The model under review builds one solid part; all positions refer to its coordinate system, in mm. Face numbers are marked on the shaded views. A direction names the side the tool comes from. Coordinates: 2 decimals unless noted, no trailing zeros. Write each loop counter-clockwise with the first axis right and the second up, starting at its lowest first coordinate (ties: lowest second). Pieces come first, ordered by that corner, then holes.
1) Mouldability with a two-part tool opening along X and no side actions: class the marked faces 1, 2, 3 and 4 as released by +X, released by -X, zero draft, split by the parting line, or undercut.
2) Machinability: for the marked faces 5 and 6, which of the approach directions +Z, -Z, +X, -X, +Y, -Y give a long, thin tool a straight path to every point of the face, cutting with its end or side? Answer none if there is none.
3) For line 1 (X direction, y = 20, z = 32); line 2 (Z direction, x = 57.5, y = 20.5); line 3 (Z direction, x = 3, y = 8.25), list the stretches that pass through material, from the lowest coordinate up.
4) Add section B-B, the plane y = 19.25. State the section outline as (x, z) points.
5) Add section C-C, the plane x = 40.5. State the section outline as (y, z) points.
6) Add section A-A, the plane x = 13.5. State the section outline as (y, z) points, then the cut area to 3 significant figures.
7) For P1, Ø10, axis at x = -8, y = 21.5, coming from the +Z side; P2, Ø2, axis at x = -6, y = 17, coming from the -Z side; P3, Ø6, axis at x = -37.69, z = -47.06, coming from the -Y side; P4, Ø0.5, axis at x = -2, z = 55.5, coming from the +Y side, all flat-tipped, find the tip position at first contact; note any pin that passes through.
8) Add section D-D, the plane z = 18.5. State the section outline as (x, y) points.
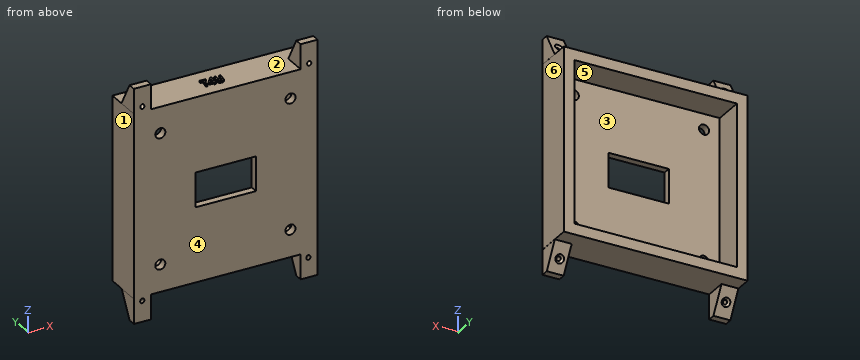
from build123d import *

# Parameters (mm, degrees)
SKETCH1_W                                            = 106
SKETCH1_H                                            = 106
SKETCH1_W_2                                          = 39.59401571
SKETCH1_H_2                                          = 22.527629628
BOSS_EXTRUDE1_DEPTH                                  = 5
SKETCH1_4_W                                          = 106
SKETCH1_4_H                                          = 106
BOSS_EXTRUDE2_DEPTH                                  = 25
SKETCH1_6_W                                          = 11.041643383
SKETCH1_6_H                                          = 16.216795515
BOSS_EXTRUDE4_DEPTH                                  = 5
SKETCH1_8_W                                          = 11.041643383
SKETCH1_8_H                                          = 16.216795515
BOSS_EXTRUDE5_DEPTH                                  = 5
SKETCH1_10_W                                         = 11.121003358
SKETCH1_10_H                                         = 16.216795515
SKETCH1_10_W_2                                       = 11.11598595
BOSS_EXTRUDE7_DEPTH                                  = 5
DRAFT1_ANGLE                                         = 1
DRAFT2_ANGLE                                         = 45
DRAFT3_ANGLE                                         = 30
DRAFT4_ANGLE                                         = 30
DRAFT6_ANGLE                                         = 30
DRAFT7_ANGLE                                         = 30
CSK_FOR_M2_5_OVAL_HEAD_MACHINE_SCREW1_D              = 2.7
CSK_FOR_M2_5_OVAL_HEAD_MACHINE_SCREW1_CSINK_D        = 5.5
CSK_FOR_M2_5_OVAL_HEAD_MACHINE_SCREW1_CSINK_ANGLE    = 90
CSK_FOR_M2_5_OVAL_HEAD_MACHINE_SCREW1_ON_D           = 2.7
CSK_FOR_M2_5_OVAL_HEAD_MACHINE_SCREW1_ON_CSINK_D     = 5.5
CSK_FOR_M2_5_OVAL_HEAD_MACHINE_SCREW1_ON_CSINK_ANGLE = 90
CSK_FOR_M2_5_OVAL_HEAD_MACHINE_SCREW_2_D             = 2.7
CSK_FOR_M2_5_OVAL_HEAD_MACHINE_SCREW_2_CSINK_D       = 5.5
CSK_FOR_M2_5_OVAL_HEAD_MACHINE_SCREW_2_CSINK_ANGLE   = 90
BOSS_EXTRUDE9_DEPTH                                  = 1
SKETCH14_R                                           = 3.296320564
CUT_EXTRUDE1_DEPTH                                   = 10


with BuildPart() as part:
    # Sketch1 → Boss-Extrude1 (new body)
    with BuildSketch(Plane(origin=(0, 0, 0), x_dir=(1, 0, 0), z_dir=(0, 1, 0))):
        with Locations((5.031290625, 4.83488638)):
            Rectangle(SKETCH1_W, SKETCH1_H)
        with Locations((5.031290625, 4.83488638)):
            Rectangle(SKETCH1_W_2, SKETCH1_H_2, mode=Mode.SUBTRACT)
    extrude(amount=BOSS_EXTRUDE1_DEPTH)

    # Sketch1<4> → Boss-Extrude2 (add)
    with BuildSketch(Plane(origin=(0, 0, 0), x_dir=(1, 0, 0), z_dir=(0, 1, 0))):
        Polygon((-54.910689044, 64.83488638), (-54.968709375, 64.83488638), (-54.968709375, -55.16511362), (-43.869045661, -55.16511362), (53.931626911, -55.16511362), (65.031290625, -55.16511362), (65.031290625, 64.83488638), (64.973270294, 64.83488638), (53.931626911, 64.83488638), (-43.869045661, 64.83488638), align=None)
        with Locations((5.031290625, 4.83488638)):
            Rectangle(SKETCH1_4_W, SKETCH1_4_H, mode=Mode.SUBTRACT)
    extrude(amount=BOSS_EXTRUDE2_DEPTH)

    # Sketch1<6> → Boss-Extrude4 (add)
    with BuildSketch(Plane(origin=(0, 0, 0), x_dir=(1, 0, 0), z_dir=(0, 1, 0))):
        with Locations((-49.389867353, 72.943284138)):
            Rectangle(SKETCH1_6_W, SKETCH1_6_H)
    extrude(amount=BOSS_EXTRUDE4_DEPTH)

    # Sketch1<8> → Boss-Extrude5 (add)
    with BuildSketch(Plane(origin=(0, 0, 0), x_dir=(1, 0, 0), z_dir=(0, 1, 0))):
        with Locations((59.452448602, 72.943284138)):
            Rectangle(SKETCH1_8_W, SKETCH1_8_H)
    extrude(amount=BOSS_EXTRUDE5_DEPTH)

    # Sketch1<10> → Boss-Extrude7 (add)
    with BuildSketch(Plane(origin=(0, 0, 0), x_dir=(1, 0, 0), z_dir=(0, 1, 0))):
        with Locations((-49.42954734, -63.273511378)):
            Rectangle(SKETCH1_10_W, SKETCH1_10_H)
        with Locations((59.489619886, -63.273511378)):
            Rectangle(SKETCH1_10_W_2, SKETCH1_10_H)
    extrude(amount=BOSS_EXTRUDE7_DEPTH)

    # Draft1
    draft1_faces = [part.faces().sort_by_distance(p)[0] for p in [
        (59.489619886, 5, 63.273511377),
    ]]
    draft(draft1_faces, Plane(origin=(0, 5, 71.381909135), x_dir=(1, 0, 0), z_dir=(0, 0, 1)), DRAFT1_ANGLE)

    # Draft2
    draft2_faces = [part.faces().sort_by_distance(p)[0] for p in [
        (59.489619886, 5.141532609, 63.273511377),
    ]]
    draft(draft2_faces, Plane(origin=(0, 5, 71.381909135), x_dir=(1, 0, 0), z_dir=(0, 0, 1)), DRAFT2_ANGLE)

    # Draft3
    draft3_faces = [part.faces().sort_by_distance(p)[0] for p in [
        (59.489619886, 13.108397758, 63.273511377),
    ]]
    draft(draft3_faces, Plane(origin=(0, 5, 71.381909135), x_dir=(1, 0, 0), z_dir=(0, 0, 1)), DRAFT3_ANGLE)

    # Draft4
    draft4_faces = [part.faces().sort_by_distance(p)[0] for p in [
        (-49.42954734, 5, 63.273511377),
    ]]
    draft(draft4_faces, Plane(origin=(0, 5, 71.381909135), x_dir=(1, 0, 0), z_dir=(0, 0, 1)), DRAFT4_ANGLE)

    # Draft6
    draft6_faces = [part.faces().sort_by_distance(p)[0] for p in [
        (-49.389867352, 5, -72.943284138),
    ]]
    draft(draft6_faces, Plane(origin=(0, 5, -81.051681895), x_dir=(-1, 0, 0), z_dir=(0, 0, -1)), DRAFT6_ANGLE)

    # Draft7
    draft7_faces = [part.faces().sort_by_distance(p)[0] for p in [
        (59.452448603, 5, -72.943284138),
    ]]
    draft(draft7_faces, Plane(origin=(0, 5, -81.051681895), x_dir=(-1, 0, 0), z_dir=(0, 0, -1)), DRAFT7_ANGLE)

    # CSK for M2.5 Oval Head Machine Screw1 (through all)
    with Locations(Plane(origin=(59.56504546, 9.768238454, 63.123077871), x_dir=(0, -0.5, 0.866025403784), z_dir=(0, 0.866025403784, 0.5))):
        with Locations((0, 0)):
            CounterSinkHole(CSK_FOR_M2_5_OVAL_HEAD_MACHINE_SCREW1_D / 2, CSK_FOR_M2_5_OVAL_HEAD_MACHINE_SCREW1_CSINK_D / 2, counter_sink_angle=CSK_FOR_M2_5_OVAL_HEAD_MACHINE_SCREW1_CSINK_ANGLE)

    # CSK for M2.5 Oval Head Machine Screw1 on (through all)
    with Locations(Plane(origin=(-49.429743133, 9.378105131, 63.798808608), x_dir=(0, -0.500000174844, 0.866025302838), z_dir=(0, 0.866025302838, 0.500000174844))):
        with Locations((0, 0)):
            CounterSinkHole(CSK_FOR_M2_5_OVAL_HEAD_MACHINE_SCREW1_ON_D / 2, CSK_FOR_M2_5_OVAL_HEAD_MACHINE_SCREW1_ON_CSINK_D / 2, counter_sink_angle=CSK_FOR_M2_5_OVAL_HEAD_MACHINE_SCREW1_ON_CSINK_ANGLE)

    # CSK for M2.5 Oval Head Machine Screw 2 (through all)
    with Locations(Plane(origin=(58.993450062, 9.334850022, -73.543501414), x_dir=(0, 0.500000174844, 0.866025302838), z_dir=(0, 0.866025302838, -0.500000174844))):
        with Locations((-1e-09, 0), (0.598054978, -108.445190593)):
            CounterSinkHole(CSK_FOR_M2_5_OVAL_HEAD_MACHINE_SCREW_2_D / 2, CSK_FOR_M2_5_OVAL_HEAD_MACHINE_SCREW_2_CSINK_D / 2, counter_sink_angle=CSK_FOR_M2_5_OVAL_HEAD_MACHINE_SCREW_2_CSINK_ANGLE)

    # Sketch12 → Boss-Extrude9 (add)
    # profile 1 of 3: a face of its own
    with BuildSketch(Plane.XY.offset(55.16511362)):
        Polygon((-3.851170658, 14.560171439), (-0.024888607, 14.560171439), (-0.162268415, 13.501838106), (-1.398686684, 13.501838106), (-2.132651027, 8.210171439), (-3.281298864, 8.210171439), (-2.548606556, 13.501838106), (-3.997454713, 13.501838106), align=None)
    # profile 2 of 3: a face of its own
    with BuildSketch(Plane.XY.offset(55.16511362)):
        Polygon((3.033084149, 14.722991952), (4.138482787, 14.722991952), (3.543170287, 10.408248363), (4.165195527, 10.408248363), (4.02781572, 9.349915029), (3.398158268, 9.349915029), (3.240425896, 8.210171439), (2.09177806, 8.210171439), (2.249510431, 9.349915029), (-0.431939889, 9.349915029), (-0.350529633, 10.451497561), align=None)
        Polygon((2.722707547, 12.786954292), (0.838823332, 10.408248363), (2.394522451, 10.408248363), align=None, mode=Mode.SUBTRACT)
    # profile 3 of 3: a face of its own
    with BuildSketch(Plane.XY.offset(55.16511362)):
        with BuildLine():
            Line((5.587330944, 14.560171439), (6.737250816, 14.560171439))
            Line((6.737250816, 14.560171439), (6.18900362, 10.632126568))
            add(Edge.make_bspline(
                [(6.18900362, 10.632126568), (6.183402023, 10.589736798), (6.172653558, 10.508398408), (6.158581474, 10.390948009), (6.147050147, 10.283246207), (6.13835648, 10.185232364), (6.130880723, 10.097032869), (6.123537243, 10.018693331), (6.12156611, 9.949475892), (6.120711369, 9.906641739), (6.120313717, 9.886713907)],
                knots=[0, 0, 0, 0, 1.370131483, 2.629037392, 3.790386942, 4.840899086, 5.781938864, 6.627066857, 7.36126714, 8, 8, 8, 8], degree=3))
            add(Edge.make_bspline(
                [(6.120313717, 9.886713907), (6.122742642, 9.828360814), (6.127388042, 9.71675862), (6.16976809, 9.558832982), (6.242605071, 9.422303405), (6.342570448, 9.306046085), (6.471150802, 9.214343156), (6.626800051, 9.151679105), (6.806028148, 9.111359223), (6.934173097, 9.107645252), (7.001834149, 9.10568426)],
                knots=[0, 0, 0, 0, 1.044998619, 1.998593913, 2.903381636, 3.798178852, 4.724466667, 5.705876195, 6.788693348, 8, 8, 8, 8], degree=3))
            add(Edge.make_bspline(
                [(7.001834149, 9.10568426), (7.057956567, 9.10757675), (7.167183867, 9.111259975), (7.325257031, 9.141736219), (7.473400904, 9.188647388), (7.56300684, 9.236972554), (7.607322931, 9.260872561)],
                knots=[0, 0, 0, 0, 1.064320597, 2.071415827, 3.046186936, 4, 4, 4, 4], degree=3))
            add(Edge.make_bspline(
                [(7.607322931, 9.260872561), (7.638661016, 9.282340052), (7.702720081, 9.326222359), (7.786339544, 9.413823207), (7.858235271, 9.520602949), (7.910381874, 9.624167973), (7.948256851, 9.722135286), (7.977464559, 9.813799465), (8.004312179, 9.922521662), (8.034401264, 10.046840649), (8.061248289, 10.18798869), (8.090077245, 10.345103027), (8.115677693, 10.519286472), (8.133525812, 10.641031997), (8.142849774, 10.704632577)],
                knots=[0, 0, 0, 0, 0.859785812, 1.75751252, 2.725816041, 3.770921983, 4.379908327, 5.106796295, 5.951169398, 6.919234109, 8.007475297, 9.209126838, 10.542031388, 12, 12, 12, 12], degree=3))
            Line((8.142849774, 10.704632577), (8.680920688, 14.560171439))
            Line((8.680920688, 14.560171439), (9.83084056, 14.560171439))
            Line((9.83084056, 14.560171439), (9.300401858, 10.761874164))
            add(Edge.make_bspline(
                [(9.300401858, 10.761874164), (9.287330457, 10.668092192), (9.262027799, 10.486555944), (9.217376218, 10.225362872), (9.170597614, 9.984815521), (9.121368674, 9.764847607), (9.067892151, 9.565539541), (9.013042193, 9.38586844), (8.953041543, 9.227611129), (8.890292597, 9.087508153), (8.821373712, 8.962161975), (8.747602604, 8.845752783), (8.666530187, 8.737141123), (8.575826106, 8.63806749), (8.481605009, 8.543048189), (8.377649998, 8.458270008), (8.267945247, 8.379873555), (8.150621707, 8.310376789), (8.026985628, 8.247221014), (7.895497152, 8.194520818), (7.758455425, 8.148438624), (7.614268415, 8.111548668), (7.463936721, 8.082329695), (7.306681889, 8.062566996), (7.143267757, 8.04903768), (7.031968043, 8.047921181), (6.975121409, 8.047350927)],
                knots=[0, 0, 0, 0, 1.689301192, 3.270025079, 4.726951413, 6.061161684, 7.290631986, 8.408026906, 9.411210366, 10.308389253, 11.14458747, 11.960942218, 12.765860093, 13.558707188, 14.355765744, 15.150991277, 15.948624031, 16.759492273, 17.581610214, 18.423095804, 19.284310986, 20.159533266, 21.076429259, 22.014764283, 22.986035413, 24, 24, 24, 24], degree=3))
            add(Edge.make_bspline(
                [(6.975121409, 8.047350927), (6.899147588, 8.048587808), (6.751454442, 8.050992305), (6.536301922, 8.076231064), (6.333976611, 8.114679105), (6.144184028, 8.169981914), (5.966590773, 8.239025973), (5.802820172, 8.326551549), (5.651359669, 8.428658918), (5.513849709, 8.546937553), (5.392382824, 8.679882671), (5.283545327, 8.822523738), (5.194999105, 8.979481857), (5.120877418, 9.146334823), (5.063065349, 9.324939947), (5.023512275, 9.515179828), (4.996651616, 9.716770462), (4.994428674, 9.855245029), (4.993290479, 9.926147)],
                knots=[0, 0, 0, 0, 1.177265359, 2.288604451, 3.35342386, 4.366487498, 5.349088925, 6.301818939, 7.238910628, 8.175748691, 9.10608431, 10.02633368, 10.950892497, 11.892606604, 12.852970325, 13.854711106, 14.901565705, 16, 16, 16, 16], degree=3))
            add(Edge.make_bspline(
                [(4.993290479, 9.926147), (4.993463542, 9.959650681), (4.993829568, 10.030510458), (4.999712409, 10.142016979), (5.007029362, 10.26504099), (5.018557194, 10.399061752), (5.03427852, 10.544419142), (5.052121268, 10.700877502), (5.072117704, 10.868893718), (5.088076227, 10.984505296), (5.096325335, 11.044265991)],
                knots=[0, 0, 0, 0, 0.71553134, 1.513337966, 2.384471215, 3.347928436, 4.386088841, 5.507247356, 6.711473103, 8, 8, 8, 8], degree=3))
            Line((5.096325335, 11.044265991), (5.587330944, 14.560171439))
        make_face()
    extrude(amount=BOSS_EXTRUDE9_DEPTH)

    # Sketch14 → Cut-Extrude1 (cut)
    with BuildSketch(Plane(origin=(0, 0, 0), x_dir=(-1, 0, 0), z_dir=(0, -1, 0))):
        with Locations(Location((37.694214755, -37.98017666, 0), (0, 0, 90))):
            Circle(SKETCH14_R)
        with Locations(Location((-47.311196673, -37.942022361, 0), (0, 0, 90))):
            Circle(SKETCH14_R)
        with Locations(Location((-47.311196673, 47.057977639, 0), (0, 0, 90))):
            Circle(SKETCH14_R)
        with Locations(Location((37.688803327, 47.057977639, 0), (0, 0, 90))):
            Circle(SKETCH14_R)
    extrude(amount=-CUT_EXTRUDE1_DEPTH, mode=Mode.SUBTRACT)


solid = part.part
Geometry results:
1. face 1: released by -X
1. face 2: undercut
1. face 3: undercut
1. face 4: zero draft
2. face 5: +Y
2. face 6: +Z, -Z, +X, +Y, -Y
3. line 1: x = -54.97 to -47.97, 58.03 to 65.03
3. line 2: z = -64.83 to -57.83, 48.17 to 55.17
3. line 3: z = -64.83 to -57.83, 48.17 to 56.17
4. outline: (-54.97, -64.83) - (65.03, -64.83) - (65.03, 55.17) - (-54.97, 55.17) - close; hole (-47.97, -57.83) - (58.03, -57.83) - (58.03, 48.17) - (-47.97, 48.17) - close
5. outline: (0, -64.83) - (25, -64.83) - (25, -57.83) - (5, -57.83) - (5, 48.17) - (25, 48.17) - (25, 55.17) - (0, 55.17) - close
6. outline: (0, -64.83) - (25, -64.83) - (25, -57.83) - (5, -57.83) - (5, -16.1) - (0, -16.1) - close; (0, 6.43) - (5, 6.43) - (5, 48.17) - (25, 48.17) - (25, 55.17) - (0, 55.17) - close
6. area: 767 mm2
7. P1: stops at z = 55.17
7. P2: stops at z = -64.83
7. P3: passes through
7. P4: stops at y = 14.56
8. outline: (-54.97, 0) - (65.03, 0) - (65.03, 25) - (58.03, 25) - (58.03, 5) - (-47.97, 5) - (-47.97, 25) - (-54.97, 25) - close
